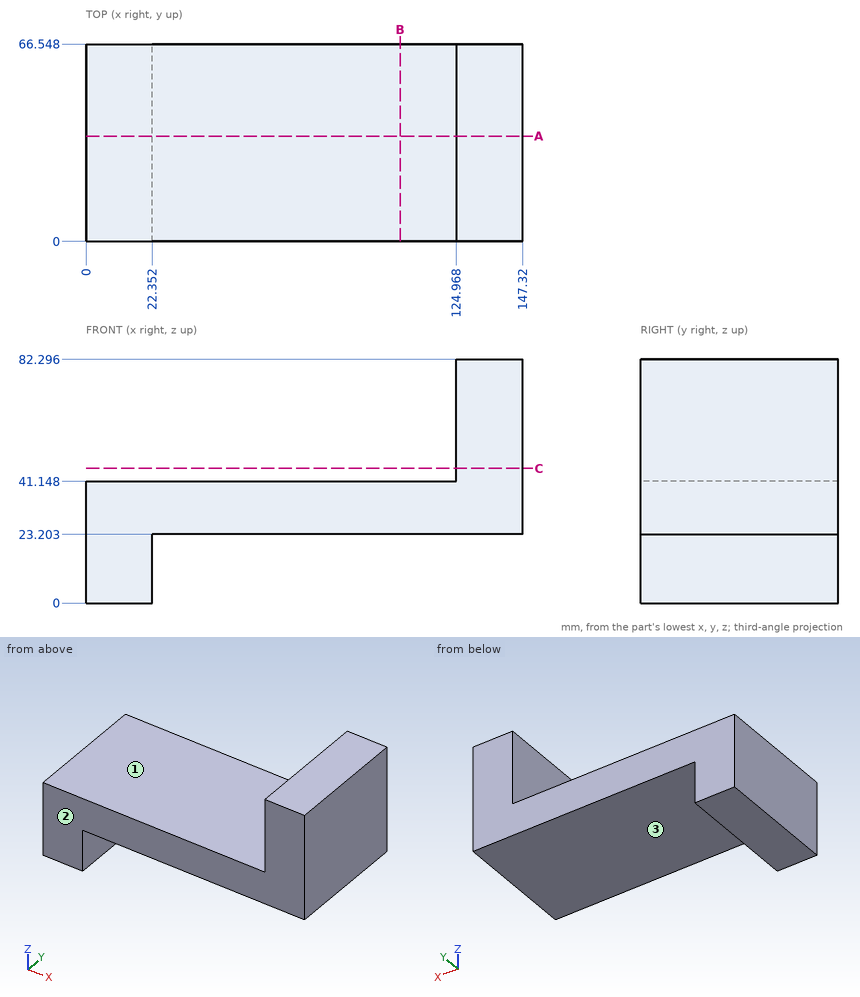
Answer from the drawing. Dimensions are ordinates in mm from the lowest x, y and z of the part. A direction names the side the tool comes from. Round coordinates to 2 decimals unless told otherwise and drop trailing zeros. Write each loop counter-clockwise with the first axis right and the second up, starting at its lowest first coordinate (ties: lowest second). Pieces come first, ordered by that corner, then holes. Notation, with made-up numbers: (-39, -32) -> (-35, -32) arc R26 ccw to (-35, -11) -> close; hole circle Ø11 at (79, 28). An arc over 180 degrees is marked (long way). Answer in a Markdown table with one row per item. Add a question column.
1) Find section A-A, the plane y = 35.5. Determine the outline of the cut face in (x, z), and give its area (3 significant figures).
2) Find section C-C, the plane z = 45.5. Determine the outline of the cut face in (x, y), and give its area (3 significant figures).
3) Given P1, Ø6, axis at x = 111.5, y = 8, coming from the +Z side; P2, Ø20, axis at x = 57.5, y = 36, coming from the -Z side; P3, Ø11.5, axis at y = 31, z = 15.5, coming from the +X side, each flat-ended and moving along its own axis, determine where each tip first touches the part or whether it passes through.
4) Find section B-B, the plane x = 106. Determine the outline of the cut face in (y, z).
5) Consider line 1 (Z direction, x = 47.5, y = 45); line 2 (X direction, y = 6, z = 9.5); line 3 (X direction, y = 35.5, z = 74). Determine where each line is inside the solid, lowest interval first.
6) Which of the six approach directions +Z, -Z, +X, -X, +Y, -Y give full straight-line access (tool end or side, diameter ignored) to the marked faces 1, 2 and 3?
Findings below:
| question | item | result |
|---|---|---|
| 1 | outline | (0, 0) -> (22.35, 0) -> (22.35, 23.2) -> (147.32, 23.2) -> (147.32, 82.3) -> (124.97, 82.3) -> (124.97, 41.15) -> (0, 41.15) -> close |
| 1 | area | 4,080 mm² |
| 2 | outline | (124.97, 0) -> (147.32, 0) -> (147.32, 66.55) -> (124.97, 66.55) -> close |
| 2 | area | 1,490 mm² |
| 3 | P1 | z = 41.15 |
| 3 | P2 | z = 23.2 |
| 3 | P3 | x = 22.35 |
| 4 | outline | (0, 23.2) -> (66.55, 23.2) -> (66.55, 41.15) -> (0, 41.15) -> close |
| 5 | line 1 | 23.2 to 41.15 |
| 5 | line 2 | 0 to 22.35 |
| 5 | line 3 | 124.97 to 147.32 |
| 6 | face 1 | +Z, -X, +Y, -Y |
| 6 | face 2 | +Z, -Z, +X, -X, -Y |
| 6 | face 3 | -Z, +X, +Y, -Y |
